from build123d import *

# Parameters (mm, degrees)
F0_R     = 20
F1_DEPTH = 8.89
F2_DEPTH = 8.89


with BuildPart() as f1:
    # F0 (on Top) → F1 (new body)
    with BuildSketch(Plane.XY):
        with Locations((-29.035902, 28.764101)):
            Circle(F0_R)
        Polygon((-29.035902, 30.496152), (-27.535902, 29.630126), (-27.535902, 27.898075), (-29.035902, 27.03205), (-30.535902, 27.898075), (-30.535902, 29.630126), align=None, mode=Mode.SUBTRACT)
    extrude(amount=F1_DEPTH)

    # F0 (on Top) → F2 (cut)
    with BuildSketch(Plane.XY):
        Polygon((-27.535902, 27.898075), (-27.535902, 29.630126), (-29.035902, 30.496152), (-30.535902, 29.630126), (-30.535902, 27.898075), (-29.035902, 27.03205), align=None)
    extrude(amount=F2_DEPTH, mode=Mode.SUBTRACT)


solid = f1.part
Design review of the part built by this model. Coordinates are the model's own, in mm. A direction names the side the tool comes from. Round coordinates to 2 decimals unless told otherwise and drop trailing zeros. Loops run counter-clockwise (first coordinate to the right, second up) from the corner with the lowest first, then second, coordinate; pieces in that order, holes last. Notation, with made-up numbers: M 37,31.25 L 56,31.25 A22 cw 56,41.25 Z; hole C -23,10.25 d8. An arc over 180 degrees is marked long. Answer as a JSON object with one key per item and string values.
Item 1: We need section A-A on x = -29.5. Give the boundary of the cut face in (y, z).
Answer sheet:
{"outline": "M 8.77,0 L 27.3,0 L 27.3,8.89 L 8.77,8.89 Z; M 30.23,0 L 48.76,0 L 48.76,8.89 L 30.23,8.89 Z"}
Item 2: Machinability: for faces 4 (the flat face through (-25, 29, 8.89)), 5 (the flat face through (-29.796, 30.057, 4.383)), which of the approach directions +Z, -Z, +X, -X, +Y, -Y give a long, thin tool a straight path to every point of the face, cutting with its end or side? Answer none if there is none.
Answer sheet:
{"face 4": "+Z, +X, -X, +Y, -Y", "face 5": "+Z, -Z"}
Item 3: The part is to be moulded in two halves that separate along Y. For faces 1 (the flat face through (-25, 29, 0)), 2 (the cylindrical face through (-33.37, 9.24, 4.38)), 3 (the flat face through (-29.78, 27.46, 4.38)), say which applies: pulls with the +Y half, pulls with the -Y half, needs draft (parallel to the pull), parting line crosses it, or undercut.
Answer sheet:
{"face 1": "needs draft", "face 2": "parting line crosses it", "face 3": "undercut"}
Item 4: We need section C-C on y = 46.5. Give the boundary of the cut face in (x, z).
Answer sheet:
{"outline": "M -38.28,0 L -19.79,0 L -19.79,8.89 L -38.28,8.89 Z"}
Item 5: We need section B-B on z = 7. Give the boundary of the cut face in (x, y).
Answer sheet:
{"outline": "C -29.04,28.76 d40; hole M -30.54,27.9 L -29.04,27.03 L -27.54,27.9 L -27.54,29.63 L -29.04,30.5 L -30.54,29.63 Z"}
Item 6: We need section D-D on x = -45.5. Give the boundary of the cut face in (y, z), and give its area (3 significant figures).
Answer sheet:
{"outline": "M 17.41,0 L 40.12,0 L 40.12,8.89 L 17.41,8.89 Z", "area": "202 mm^2"}
Item 7: Clearance check with flat-ended pins moving along their axes: P1, Ø1.5, axis at y = 18, z = 4, coming from the -X side; P2, Ø1.5, axis at x = -40, y = 39.5, coming from the -Z side; P3, Ø1, axis at x = -33.5, z = 2, coming from the +Y side; P4, Ø3, axis at y = 23, z = 3, coming from the -X side. State where each tip first meets the part, or that it passes through.
Answer sheet:
{"P1": "stops at x = -46.35", "P2": "stops at z = 0", "P3": "stops at y = 48.37", "P4": "stops at x = -48.58"}
Item 8: Wall thickness on L1, parallel to X at y = 30, z = 3.5; L2, parallel to Y at x = -44.5, z = 6.75; L3, parallel to Y at x = -35, z = 4.75: over which ranges is each line inside the solid? List them lowest first. Write a range as from..to.
Answer sheet:
{"L1": "x = -49..-29.9, -28.18..-9.07", "L2": "y = 16.08..41.45", "L3": "y = 9.67..47.85"}
